```python
from build123d import *

# Parameters (mm, degrees)
F0_R     = 7.5
F1_DEPTH = 7.1
F2_R     = 1.75
F3_DEPTH = 4
F4_R     = 6


with BuildPart() as f1:
    # F0 (on Top) → F1 (new body)
    with BuildSketch(Plane.XY):
        Circle(F0_R)
    extrude(amount=F1_DEPTH)

    # F2 (on face) → F3 (cut)
    with BuildSketch(Plane(origin=(0, 0, 0), x_dir=(1, 0, 0), z_dir=(0, 0, -1))):
        Circle(F2_R)
    extrude(amount=-F3_DEPTH, mode=Mode.SUBTRACT)

    # F4
    f4_edges = [f1.edges().sort_by_distance(p)[0] for p in [
        (-7.5, 0, 7.1),
    ]]
    fillet(f4_edges, radius=F4_R)


solid = f1.part
```
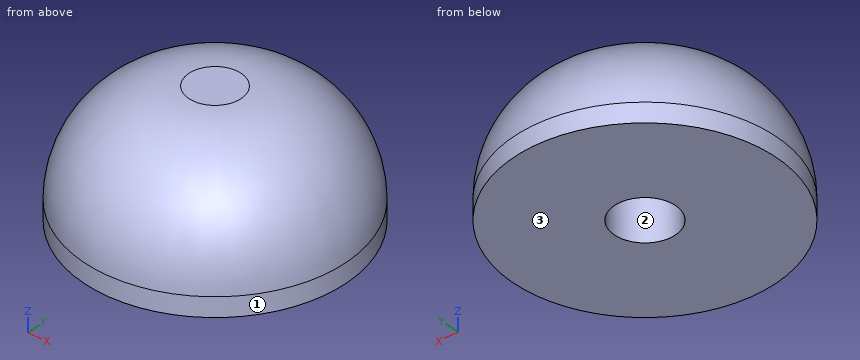
Geometry check sheet. Reference: the model listing, model coordinates, mm. Face numbers are marked on the shaded views. Coordinates: 2 decimals unless noted, no trailing zeros. Put each result on its own line as item: value.
1) Gauge pin test, flat ends, axial feed: pin 1 Ø3 at (x, y) = (0, -3) entering from +Z; pin 2 Ø2 at (x, y) = (-3.5, -3) entering from +Z; pin 3 Ø1.5 at (y, z) = (3.5, 4) entering from +X; pin 4 Ø1 at (x, z) = (-1, 3.5) entering from -Y. Record the tip position at first contact, or that the pin passes through.
Result set:
pin 1: stops at z = 7.1
pin 2: stops at z = 6.72
pin 3: stops at x = 6.35
pin 4: stops at y = -7.13
2) Thickness scan on line 1 (X direction, y = 0, z = 1.15); line 2 (Y direction, x = 0, z = 3.15). Record the ranges inside material, lowest first.
Result set:
line 1: x = -7.5 to -1.75, 1.75 to 7.5
line 2: y = -7.14 to -1.75, 1.75 to 7.14
3) Release check for a two-part mould opening along X. For the marked faces 1, 2 and 3 record: released by +X, released by -X, zero draft, split by the parting line, or undercut.
Result set:
face 1: split by the parting line
face 2: undercut
face 3: zero draft
